Part model, mm, in its own coordinate system. Face numbers are marked on the shaded views. A direction names the side the tool comes from. Round coordinates to 2 decimals unless told otherwise and drop trailing zeros. Write each loop counter-clockwise with the first axis right and the second up, starting at its lowest first coordinate (ties: lowest second). Pieces come first, ordered by that corner, then holes.
```python
from build123d import *

# Parameters (mm, degrees)
IZIM1_W                     = 140
IZIM1_H                     = 65
Y_KSEKLIK_EKSTR_ZYON1_DEPTH = 25
BO_ALTMA3_T                 = 6
IZIM2_R                     = 2.25
KES_EKSTR_ZYON1_DEPTH       = 25
IZIM3_W                     = 13.33242511
IZIM3_H                     = 17.74072696
KES_EKSTR_ZYON2_DEPTH       = 25
RADYUS1_R                   = 2
Y_KSEKLIK_EKSTR_ZYON2_START = 25
IZIM4_R                     = 2.25
Y_KSEKLIK_EKSTR_ZYON2_DEPTH = 25
IZIM5_R                     = 1
KES_EKSTR_ZYON3_DEPTH       = 20
KES_EKSTR_ZYON4_START       = -20
IZIM6_R                     = 1
KES_EKSTR_ZYON4_DEPTH       = 20


# Read off the part's stored shape, not the designer's step: M2 Dişli Delik1
with BuildPart() as part:
    # Çizim1 → Yükseklik-Ekstrüzyon1 (new body)
    with BuildSketch(Plane.XY):
        Rectangle(IZIM1_W, IZIM1_H)
    extrude(amount=Y_KSEKLIK_EKSTR_ZYON1_DEPTH)

    # İç Boşaltma3
    bo_altma3_openings = [part.faces().sort_by_distance(p)[0] for p in [
        (0, 0, 0),
    ]]
    offset(amount=BO_ALTMA3_T, openings=bo_altma3_openings, kind=Kind.INTERSECTION)

    # Çizim2 → Kes-Ekstrüzyon1 (cut)
    with BuildSketch(Plane(origin=(0, 0, 0), x_dir=(-1, 0, 0), z_dir=(0, 0, -1))):
        with Locations((-73, -35.5)):
            Circle(IZIM2_R)
        with Locations(Location((73, -35.5, 0), (0, 0, 180))):
            Circle(IZIM2_R)
        with Locations(Location((-73, 35.5, 0), (0, 0, 180))):
            Circle(IZIM2_R)
        with Locations((73, 35.5)):
            Circle(IZIM2_R)
    extrude(amount=-KES_EKSTR_ZYON1_DEPTH, mode=Mode.SUBTRACT)

    # Çizim3 → Kes-Ekstrüzyon2 (cut)
    with BuildSketch(Plane.ZY.offset(-70)):
        with Locations((15.822558672, 0)):
            Rectangle(IZIM3_W, IZIM3_H)
    extrude(amount=-KES_EKSTR_ZYON2_DEPTH, mode=Mode.SUBTRACT)

    # Radyus1
    radyus1_edges = [part.edges().sort_by_distance(p)[0] for p in [
        (76, -38.5, 15.5),
        (-76, -38.5, 15.5),
        (-76, 38.5, 15.5),
        (76, 38.5, 15.5),
    ]]
    fillet(radyus1_edges, radius=RADYUS1_R)

    # Çizim4 → Yükseklik-Ekstrüzyon2 (add)
    with BuildSketch(Plane(origin=(0, 0, 25), x_dir=(-1, 0, 0), z_dir=(0, 0, -1)).offset(Y_KSEKLIK_EKSTR_ZYON2_START)):
        with Locations((73, 35.5)):
            Circle(IZIM4_R)
        with Locations((73, -35.5)):
            Circle(IZIM4_R)
        with Locations((-73, 35.5)):
            Circle(IZIM4_R)
        with Locations((-73, -35.5)):
            Circle(IZIM4_R)
    extrude(amount=-Y_KSEKLIK_EKSTR_ZYON2_DEPTH)

    # Çizim5 → Kes-Ekstrüzyon3 (cut)
    with BuildSketch(Plane(origin=(76, 0, 0), x_dir=(0, 0, -1), z_dir=(1, 0, 0))):
        with Locations((-3, 28.5)):
            Circle(IZIM5_R)
        with Locations(Location((-3, -28.5, 0), (0, 0, 180))):
            Circle(IZIM5_R)
    extrude(amount=-KES_EKSTR_ZYON3_DEPTH, mode=Mode.SUBTRACT)

    # Çizim6 → Kes-Ekstrüzyon4 (cut)
    with BuildSketch(Plane.ZY.offset(76).offset(KES_EKSTR_ZYON4_START)):
        with Locations(Location((3, 28.5, 0), (0, 0, 180))):
            Circle(IZIM6_R)
        with Locations((3, -28.5)):
            Circle(IZIM6_R)
    extrude(amount=KES_EKSTR_ZYON4_DEPTH, mode=Mode.SUBTRACT)

    # M2 Dişli Delik1 outline → M2 Dişli Delik1 (revolve, cut)
    with BuildSketch(Plane(origin=(0, 28.5, 3), x_dir=(0, 1, 0), z_dir=(0, 0, -1))):
        Polygon((1, 76), (1, 75.97124079), (1.025, 76), align=None)
        Polygon((1.025, -76), (1, -75.97124079), (1, -76), align=None)
    revolve(axis=Axis((0, 28.5, 3), (1, 0, 0)), mode=Mode.SUBTRACT)

    # M2 Di_li Delik1 2 outline → M2 Di_li Delik1 2 (revolve, cut)
    with BuildSketch(Plane(origin=(0, -28.5, 3), x_dir=(0, 1, 0), z_dir=(0, 0, -1))):
        Polygon((1, 76), (1, 75.97124079), (1.025, 76), align=None)
        Polygon((1.025, -76), (1, -75.97124079), (1, -76), align=None)
    revolve(axis=Axis((0, -28.5, 3), (1, 0, 0)), mode=Mode.SUBTRACT)


solid = part.part
```
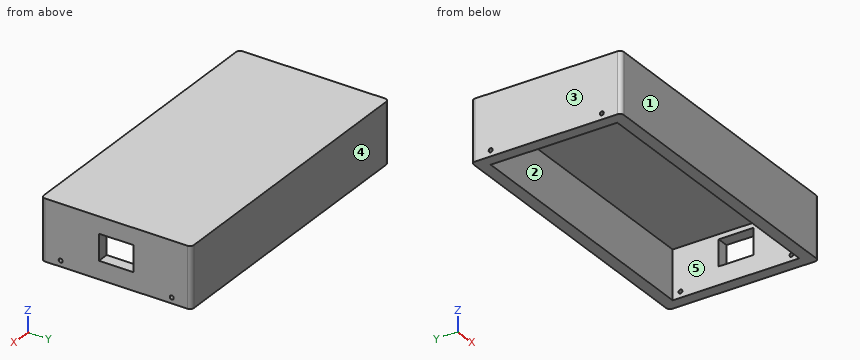
Q1. Drop flat-ended pins along their axis: pin 1 (1.6 mm diameter, centred on y = -28.5, z = 3, fed in from -X); pin 2 (10 mm diameter, centred on x = -40, y = -22.5, fed in from -Z). Give the stop position or say it passes through.
Values follow:
pin 1: passes through
pin 2: stops at z = 25
Q2. Cut at C-C on x = -8.5. Write the cut outline in (y, z), plus the area to 3 significant figures.
Values follow:
outline: (-38.5, 0) - (-32.5, 0) - (-32.5, 25) - (32.5, 25) - (32.5, 0) - (38.5, 0) - (38.5, 31) - (-38.5, 31) - close
area: 762 mm2
Q3. Which spindle directions (+Z, -Z, +X, -X, +Y, -Y) get a long thin tool onto all of the face, cutting with end or side? Do the marked faces 4 and 5. Say none if no direction does.
Values follow:
face 4: +Z, -Z, +X, -X, +Y
face 5: -Z
Q4. Cut at A-A on y = -6. Write the cut outline in (x, z).
Values follow:
outline: (-76, 0) - (-70, 0) - (-70, 25) - (70, 25) - (70, 22.49) - (76, 22.49) - (76, 31) - (-76, 31) - close; (70, 0) - (76, 0) - (76, 9.16) - (70, 9.16) - close
Q5. Cut at B-B on z = 7. Write the cut outline in (x, y).
Values follow:
outline: (-76, -36.5) arc R2 ccw to (-74, -38.5) - (74, -38.5) arc R2 ccw to (76, -36.5) - (76, 36.5) arc R2 ccw to (74, 38.5) - (-74, 38.5) arc R2 ccw to (-76, 36.5) - close; hole (-70, -32.5) - (70, -32.5) - (70, 32.5) - (-70, 32.5) - close
Q6. Wall check: L1, parallel to Z at x = 74.5, y = -28.5; L2, parallel to Y at x = -55, z = 14; L3, parallel to X at y = 29.5, z = 24. Give the ranges that are in metal, low to high.
Values follow:
L1: z = 0 to 2, 4 to 31
L2: y = -38.5 to -32.5, 32.5 to 38.5
L3: x = -76 to -70, 70 to 76
Q7. Cut at D-D on z = 21. Write the cut outline in (x, y).
Values follow:
outline: (-76, -36.5) arc R2 ccw to (-74, -38.5) - (74, -38.5) arc R2 ccw to (76, -36.5) - (76, -8.87) - (70, -8.87) - (70, -32.5) - (-70, -32.5) - (-70, 32.5) - (70, 32.5) - (70, 8.87) - (76, 8.87) - (76, 36.5) arc R2 ccw to (74, 38.5) - (-74, 38.5) arc R2 ccw to (-76, 36.5) - close
Q8. Mould opens along Y. For the marked faces 1, 2 and 3 say: +Y half, -Y half, draft (parallel to the pull), parting line (faces both ways), or undercut.
Values follow:
face 1: -Y half
face 2: undercut
face 3: draft
